Geometry: final body of the model. Coordinates: model frame, mm. A direction names the side the tool comes from. Give positions to 0.01 mm unless a question says otherwise; leave off trailing zeros. Write each loop counter-clockwise with the first axis right and the second up, starting at its lowest first coordinate (ties: lowest second). Pieces come first, ordered by that corner, then holes.
from build123d import *

# Parameters (mm, degrees)
SKETCH1_R            = 17.5
SKETCH1_R_2          = 10
BOSS_EXTRUDE1_DEPTH  = 20
SKETCH2_R            = 15
SKETCH2_R_2          = 10
BOSS_EXTRUDE2_DEPTH  = 100
BOSS_EXTRUDE6_DEPTH  = 20
BOSS_EXTRUDE7_DEPTH  = 20
SKETCH10_R           = 12.5
BOSS_EXTRUDE9_DEPTH  = 20
BOSS_EXTRUDE10_DEPTH = 20
SKETCH16_R           = 12.5
CUT_EXTRUDE1_DEPTH   = 20


with BuildPart() as part:
    # Sketch1 → Boss-Extrude1 (new body)
    with BuildSketch(Plane.XY):
        with BuildLine():
            Line((0, 138), (0, 0))
            Line((0, 0), (582.5, 0))
            Line((582.5, 0), (582.5, 51.183651))
            Line((582.5, 51.183651), (572.5, 51.183651))
            Line((572.5, 51.183651), (374.6494, 86.07005))
            Line((374.6494, 86.07005), (244.94, 310.733321))
            ThreePointArc((244.94, 310.733321), (200.912249, 330.84879), (153, 337.740187))
            Line((153, 337.740187), (153, 281.918848))
            Line((153, 281.918848), (4.984782, 149.16671))
            ThreePointArc((4.984782, 149.16671), (1.302769, 144.114398), (0, 138))
        make_face()
        with Locations((153, 167.740187)):
            Circle(SKETCH1_R, mode=Mode.SUBTRACT)
        with Locations((15, 138)):
            Circle(SKETCH1_R_2, mode=Mode.SUBTRACT)
    extrude(amount=BOSS_EXTRUDE1_DEPTH)

    # Sketch2 → Boss-Extrude2 (add)
    with BuildSketch(Plane.XY.offset(20)):
        with Locations((15, 138)):
            Circle(SKETCH2_R)
        with Locations((15, 138)):
            Circle(SKETCH2_R_2, mode=Mode.SUBTRACT)
    extrude(amount=-BOSS_EXTRUDE2_DEPTH)

    # Sketch4 → Boss-Extrude6 (add)
    with BuildSketch(Plane.XY.offset(20)):
        with BuildLine():
            Line((257.460496, 337.740187), (153, 337.740187))
            ThreePointArc((153, 337.740187), (200.912249, 330.84879), (244.94, 310.733321))
            Line((244.94, 310.733321), (374.6494, 86.07005))
            Line((374.6494, 86.07005), (426.173106, 76.98503))
            Line((426.173106, 76.98503), (290.842774, 311.384043))
            Line((290.842774, 311.384043), (257.460496, 311.384043))
            Line((257.460496, 311.384043), (257.460496, 337.740187))
        make_face()
    extrude(amount=-BOSS_EXTRUDE6_DEPTH)

    # Sketch9 → Boss-Extrude7 (add)
    with BuildSketch(Plane.XY.offset(20)):
        Polygon((320.509364, 260), (522.5, 260), (582.5, 260), (582.5, 51.183651), (572.5, 51.183651), (522.5, 60), (426.173106, 76.98503), align=None)
    extrude(amount=-BOSS_EXTRUDE7_DEPTH)



with BuildPart() as body_2:
    # Sketch10 → Boss-Extrude9 (new body)
    with BuildSketch(Plane.XY.offset(20)):
        Polygon((270.460496, 418.251615), (270.460496, 364.320187), (317.180522, 364.320187), (324.460496, 364.320187), (324.460496, 418.251615), align=None)
        with Locations((297.460496, 398.384043)):
            Circle(SKETCH10_R, mode=Mode.SUBTRACT)
        Polygon((270.460496, 364.320187), (257.460496, 364.320187), (257.460496, 337.740187), (257.460496, 311.384043), (290.842774, 311.384043), (317.180522, 311.384043), (317.180522, 321.223855), (317.180522, 364.320187), align=None)
        with Locations((297.460496, 346.134043)):
            Circle(SKETCH10_R, mode=Mode.SUBTRACT)
        Polygon((324.460496, 364.320187), (317.180522, 364.320187), (317.180522, 321.223855), (347.650509, 321.223855), (378.120496, 321.223855), (378.120496, 364.320187), align=None)
        with Locations((351.710496, 341.56)):
            Circle(SKETCH10_R, mode=Mode.SUBTRACT)
        Polygon((347.650509, 321.223855), (317.180522, 321.223855), (317.180522, 311.384043), (317.180522, 265.765724), (320.509364, 260), (378.120496, 260), (378.120496, 321.223855), align=None)
        with Locations((351.710496, 301)):
            Circle(SKETCH10_R, mode=Mode.SUBTRACT)
    extrude(amount=-BOSS_EXTRUDE9_DEPTH)


with BuildPart() as part_1:
    add(part.part)

    add(body_2.part)  # Boss-Extrude10 merges body 2
    # Sketch14 → Boss-Extrude10 (add)
    with BuildSketch(Plane(origin=(0, 0, 0), x_dir=(-1, 0, 0), z_dir=(0, 0, -1))):
        Polygon((-320.509364, 260), (-426.173106, 76.98503), (-522.5, 60), (-572.5, 60), (-582.5, 60), (-582.5, 338.045557), (-522.5, 338.045557), (-381.119364, 338.045557), (-381.119364, 260), align=None)
    extrude(amount=-BOSS_EXTRUDE10_DEPTH)

    # Sketch16 → Cut-Extrude1 (cut)
    with BuildSketch(Plane.XY.offset(20)):
        with Locations((544.895661, 294.516191)):
            Circle(SKETCH16_R)
        with Locations((544.895661, 244.516191)):
            Circle(SKETCH16_R)
    extrude(amount=-CUT_EXTRUDE1_DEPTH, mode=Mode.SUBTRACT)


solid = part_1.part
Q1. Section A-A on x = 15. Output: boundary loops of the cut face in (y, z), plus the area to 3 significant figures.
Filled sheet:
outline: (0, 0) - (123, 0) - (123, -80) - (128, -80) - (128, 20) - (0, 20) - close; (148, -80) - (153, -80) - (153, 0) - (158.15, 0) - (158.15, 20) - (148, 20) - close
area: 3,560 mm2
Q2. Section C-C on y = 35.5. Output: boundary loops of the cut face in (x, z), plus the area to 4 significant figures.
Filled sheet:
outline: (0, 0) - (582.5, 0) - (582.5, 20) - (0, 20) - close
area: 11,650 mm2
Q3. Section D-D on x = 371. Output: boundary loops of the cut face in (y, z).
Filled sheet:
outline: (0, 0) - (364.32, 0) - (364.32, 20) - (0, 20) - close
Q4. Ray query, line 1 along X through (y, z) = (341, 15); line 2 along Z through (x, y) = (440.5, 235); line 3 along X through (y, z) = (286.5, 3). Return the intervals inside material, ascending.
Filled sheet:
line 1: x = 257.46 to 286.06, 308.86 to 339.22, 364.2 to 378.12
line 2: z = 0 to 20
line 3: x = 153 to 305.21, 317.18 to 378.12, 381.12 to 535.3, 554.49 to 582.5
Q5. Pull-direction query (Y, two-part tool) for faces 1 (the cylindrical face through (139.113, 157.092, 9.86)), 2 (the flat face through (352, 364.32, 10)), 3 (the flat face through (381.119, 300, 10)); classes: released by +Y, released by -Y, zero draft, split by the parting line, or undercut.
Filled sheet:
face 1: undercut
face 2: released by +Y
face 3: zero draft
Q6. Section B-B on y = 301. Output: boundary loops of the cut face in (x, z).
Filled sheet:
outline: (153, 0) - (296.84, 0) - (296.84, 20) - (153, 20) - close; (317.18, 0) - (339.21, 0) - (339.21, 20) - (317.18, 20) - close; (364.21, 0) - (378.12, 0) - (378.12, 20) - (364.21, 20) - close; (381.12, 0) - (534.21, 0) - (534.21, 20) - (381.12, 20) - close; (555.58, 0) - (582.5, 0) - (582.5, 20) - (555.58, 20) - close
Q7. Access query for faces 4 (the flat face through (480, 338.046, 10)), 5 (the flat face through (25, 135, -80)), 6 (the flat face through (378.12, 311, 10)), 7 (the flat face through (153, 310, 10)), 8 (the cylindrical face through (363.257, 296.212, 10.14)). Directions: +Z, -Z, +X, -X, +Y, -Y. A direction counts if a zero-diameter tool reaches every point of the face in a straight line with its end or side. Return the directions, or none.
Filled sheet:
face 4: +Z, -Z, +X, +Y
face 5: -Z, +X, -X, +Y, -Y
face 6: +Z, -Z, +Y
face 7: +Z, -Z, -X, +Y
face 8: +Z, -Z
Q8. Pin query (flat end, axial travel): P1, Ø16, axis at y = 306.5, z = 9, coming from the -X side; P2, Ø10, axis at x = 228, y = 194.5, coming from the -Z side; P3, Ø14.5, axis at x = 261.5, z = 11.5, coming from the +Y side. Return the tip coordinate at first contact, or that it passes through.
Filled sheet:
P1: stops at x = 153
P2: stops at z = 0
P3: stops at y = 364.32
